Geometry: see drawing. Coordinates: mm, zero at the bounding-box minimum. A direction names the side the tool comes from. Round coordinates to 2 decimals unless told otherwise and drop trailing zeros. Order: outer loops, then holes, each group sorted by start corner. A loop starts at its lowest first (then second) coordinate and runs counter-clockwise, first axis right, second up. Notation, with made-up numbers: (88.25, 33.25) - (126.25, 33.25) arc R28 ccw to (126.25, 55.25) - close; hole circle Ø8 at (40, 18.5). An arc over 180 degrees is marked (long way). Put each result on its own line as item: value. Start each with the question number.
1) Contact query for flat-ended pins moving along their axis: P1, Ø0.6, axis at x = 29, y = 4.5, coming from the +Z side; P2, Ø1, axis at x = 8, z = 4.5, coming from the +Y side (3 decimals); P3, Ø5.5, axis at y = 11.66, z = 5, coming from the -X side. Output: stop coordinate, or through.
2) Section A-A on z = 5. Output: boundary loops of the cut face in (x, y) (3 decimals), then the cut area to 3 significant figures.
3) Access query for the marked faces 1 and 2. Directions: +Z, -Z, +X, -X, +Y, -Y. A direction counts if a zero-diameter tool reaches every point of the face in a straight line with its end or side. Return the directions, or none.
4) Mould query, pull axis Z, two halves, no side actions, for the marked faces 3, 4 and 5. Classes: +Z half, -Z half, draft (parallel to the pull), parting line (faces both ways), or undercut.
5) Section D-D on y = 23.5. Output: boundary loops of the cut face in (x, z), then the cut area to 3 significant figures.
6) Section C-C on x = 4. Output: boundary loops of the cut face in (y, z) (3 decimals).
7) Line query: probe 1 along X at (y, z) = (5, 4.75); probe 2 along Y at (x, z) = (6.5, 4) (3 decimals); probe 3 along Z at (x, y) = (16.5, 10.5). Output: solid intervals per line, ascending. Write a range as [from, to].
8) Section B-B on x = 30. Output: boundary loops of the cut face in (y, z) (3 decimals), then the cut area to 3 significant figures.
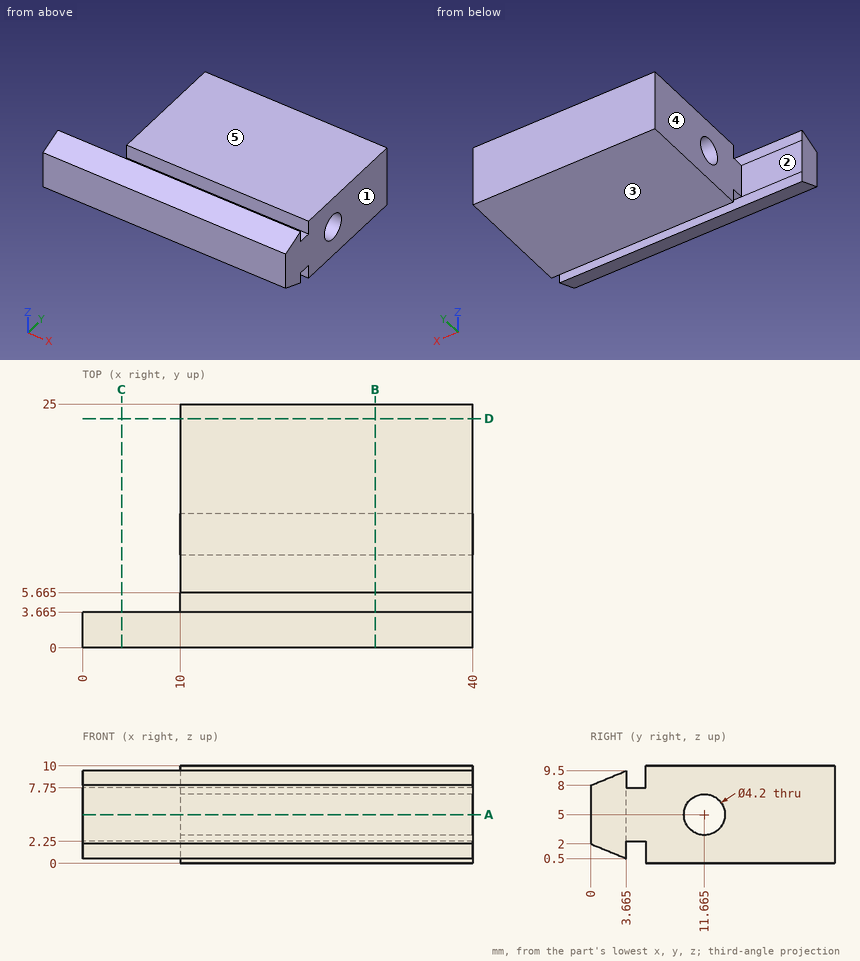
Answer sheet:
1. P1: z = 7.75
1. P2: y = 3.665
1. P3: x = 10
2. outline: (0, 0) - (40, 0) - (40, 9.565) - (10, 9.565) - (10, 3.665) - (0, 3.665) - close; (10, 13.765) - (40, 13.765) - (40, 25) - (10, 25) - close
2. area: 661 mm^2
3. face 1: +Z, -Z, +X, +Y, -Y
3. face 2: +Z, -Z, -X, +Y
4. face 3: -Z half
4. face 4: draft
4. face 5: +Z half
5. outline: (10, 0) - (40, 0) - (40, 10) - (10, 10) - close
5. area: 300 mm^2
6. outline: (0, 2) - (3.665, 0.5) - (3.665, 9.5) - (0, 8) - close
7. probe 1: [10, 40]
7. probe 2: [0, 3.665]
7. probe 3: [0, 3.25], [6.75, 10]
8. outline: (0, 2) - (3.665, 0.5) - (3.665, 2.25) - (5.665, 2.25) - (5.665, 0) - (25, 0) - (25, 10) - (5.665, 10) - (5.665, 7.75) - (3.665, 7.75) - (3.665, 9.5) - (0, 8) - close; hole circle Ø4.2 at (11.665, 5)
8. area: 218 mm^2
